```python
from build123d import *

# Parameters (mm, degrees)
SKETCH1_R           = 70.25
SKETCH1_R_2         = 48
BOSS_EXTRUDE1_DEPTH = 3
SKETCH2_W           = 13.3
SKETCH2_H           = 3
CUT_EXTRUDE1_DEPTH  = 3
CIRPATTERN1_COUNT   = 12


with BuildPart() as part:
    # Sketch1 → Boss-Extrude1 (new body)
    with BuildSketch(Plane(origin=(0, 0, 0), x_dir=(1, 0, 0), z_dir=(0, 1, 0))):
        with Locations(Location((0, 0, 0), (0, 0, 270))):
            Circle(SKETCH1_R)
        with Locations(Location((0, 0, 0), (0, 0, 270))):
            Circle(SKETCH1_R_2, mode=Mode.SUBTRACT)
    extrude(amount=BOSS_EXTRUDE1_DEPTH)

    # Sketch2 → Cut-Extrude1 (cut)
    with BuildSketch(Plane(origin=(0, 3, 0), x_dir=(1, 0, 0), z_dir=(0, 1, 0))):
        with Locations((-63.6, 0)):
            Rectangle(SKETCH2_W, SKETCH2_H)
    cut_extrude1 = extrude(amount=-CUT_EXTRUDE1_DEPTH, mode=Mode.SUBTRACT)

    # CirPattern1: Cut-Extrude1 ×12 about axis
    cirpattern1_axis = Axis((0, 0, 0), (0, 1, 0))
    for i in range(1, CIRPATTERN1_COUNT):
        add(cut_extrude1.rotate(cirpattern1_axis, i * 360 / CIRPATTERN1_COUNT), mode=Mode.SUBTRACT)


solid = part.part
```
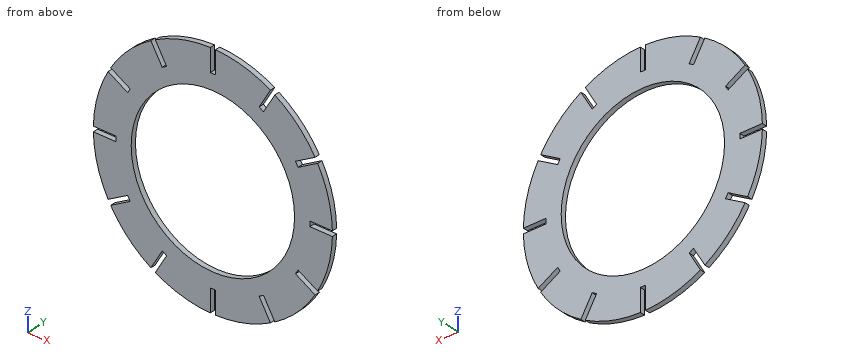
Verification items for the finished model (mm, model axes). Give positions to 0.01 mm unless a question says otherwise; leave off trailing zeros. Order: outer loops, then holes, each group sorted by start corner. A loop starts at its lowest first (then second) coordinate and runs counter-clockwise, first axis right, second up. Notation, with made-up numbers: M 46.5,17 L 54.5,17 A27 ccw 54.5,45 Z; hole C 66.5,42 d6. An arc over 180 degrees is marked long. Answer in a Markdown table with one row per item. Add a question column.
Item 1: Scan lines: probe 1 along Z at (x, y) = (1, 0.65); probe 2 along Z at (x, y) = (-57.5, 2.8); probe 3 along X at (y, z) = (1.05, 0). Record each from-to range of solid material in increasing order. Write a range as from..to.
Item 2: Section check A-A, the plane x = 25.5. Enter the section's corners in (y, z).
Item 3: Section check B-B, the plane z = -45. Enter the section's corners in (x, y) (3 decimals), and give its area (3 significant figures).
Item 4: Gauge pin test, flat ends, axial feed: pin 1 (0.9 mm diameter, centred on x = -61, y = 1, fed in from +Z); pin 2 (1 mm diameter, centred on x = -20, y = 1.5, fed in from +Z); pin 3 (0.9 mm diameter, centred on y = 2, z = 0, fed in from +X). Record the tip position at first contact, or that the pin passes through.
Filled sheet:
| question | item | result |
|---|---|---|
| 1 | probe 1 | z = -56.95..-47.99, 47.99..56.95 |
| 1 | probe 2 | z = -40.36..-34.93, -31.47..-1.5, 1.5..31.47, 34.93..40.36 |
| 1 | probe 3 | x = -56.95..-48, 48..56.95 |
| 2 | outline | M 0,-65.46 L 3,-65.46 L 3,-40.67 L 0,-40.67 Z; M 0,40.67 L 3,40.67 L 3,65.46 L 0,65.46 Z |
| 3 | outline | M -53.945,0 L -16.703,0 L -16.703,3 L -53.945,3 Z; M 16.703,0 L 53.945,0 L 53.945,3 L 16.703,3 Z |
| 3 | area | 223 mm^2 |
| 4 | pin 1 | stops at z = 33.75 |
| 4 | pin 2 | stops at z = 67.49 |
| 4 | pin 3 | stops at x = 56.95 |
